from build123d import *

# Parameters (mm, degrees)
F0_W     = 20
F0_H     = 80
F1_DEPTH = 5
F3_W     = 5
F3_H     = 5
F3_R     = 0.75
F4_DEPTH = 10
F2_W     = 4.293
F2_H     = 4.31325
F2_R     = 0.75
F5_DEPTH = 5
F6_W     = 10
F6_H     = 20
F7_DEPTH = 30


with BuildPart() as f1:
    # F0 (on Front) → F1 (new body)
    with BuildSketch(Plane.XZ):
        Rectangle(F0_W, F0_H)
    extrude(amount=F1_DEPTH)

    # F3 (on Front) → F4 (join)
    with BuildSketch(Plane.XZ):
        with Locations((-0.917875, 18.532625)):
            Rectangle(F3_W, F3_H)
        with Locations((-0.917875, 18.532625)):
            Circle(F3_R, mode=Mode.SUBTRACT)
    extrude(amount=F4_DEPTH)

    # F2 (on face) → F5 (join)
    with BuildSketch(Plane.XZ.offset(5)):
        with Locations((-7.8535, -37.843375)):
            Rectangle(F2_W, F2_H)
        with Locations((-7.8535, -37.843375)):
            Circle(F2_R, mode=Mode.SUBTRACT)
    extrude(amount=F5_DEPTH)

    # F6 (on Front) → F7 (join)
    with BuildSketch(Plane.XZ):
        with Locations((15, 0)):
            Rectangle(F6_W, F6_H)
        Polygon((20, -10), (10, -10), (20, -20), align=None)
        Polygon((20, 20), (10, 10), (20, 10), align=None)
    extrude(amount=F7_DEPTH)


solid = f1.part
Source: CAD feature listing. Evaluate the final solid. Frame: model axes, mm. A direction names the side the tool comes from. Round coordinates to 2 decimals unless told otherwise and drop trailing zeros. Loops run counter-clockwise (first coordinate to the right, second up) from the corner with the lowest first, then second, coordinate; pieces in that order, holes last.
Q1. First-contact query: P1, Ø1.5, axis at x = -1, y = -6.5, coming from the -Z side; P2, Ø2.5, axis at y = -7.5, z = 17.5, coming from the -X side; P3, Ø2, axis at y = -6.5, z = -37, coming from the +X side. Flat tips, straight axial feed; report the tip coordinate or a pass-through.
Q2. Section A-A, the plane z = 14. Return loops of the section in (x, y), plus the area to 3 significant figures.
Q3. Mould query, pull axis X, two halves, no side actions, for faces 1 (the face through (10, -2, -25)), 2 (the face through (-1, -7, 21.033)), 3 (the face through (20, -15, 0)), 4 (the face through (10, -17, 0)). Classes: pulls with the +X half, pulls with the -X half, needs draft (parallel to the pull), parting line crosses it, or undercut.
Q4. Ray query, line 1 (X direction, y = -21.75, z = -7.5); line 2 (X direction, y = -7, z = -36); line 3 (Y direction, x = 9, z = -10.5). Return the intervals inside material, ascending.
Q5. Access query for faces 5 (the face through (-8, -7, -35.687)), 6 (the face through (1.582, -7, 18)), 7 (the face through (-5.707, -7, -38)), 8 (the face through (-7.51, -7.46, -38.51)), 9 (the face through (15, -15, -15)). Directions: +Z, -Z, +X, -X, +Y, -Y. A direction counts if a zero-diameter tool reaches every point of the face in a straight line with its end or side. Return the directions, or none.
Q6. Section D-D, the plane x = 2.5. Return loops of the section in (y, z), plus the area to 3 significant figures.
Q7. Section B-B, the plane y = -3.25. Return loops of the section in (x, z), plus the area to 3 significant figures.
Q8. Section C-C, the plane z = -6. Return loops of the section in (x, y).
Solutions:
1. P1: stops at z = 16.03
1. P2: stops at x = -3.42
1. P3: stops at x = -5.71
2. outline: (-10, -5) - (10, -5) - (10, 0) - (-10, 0) - close; (14, -30) - (20, -30) - (20, 0) - (14, 0) - close
2. area: 280 mm2
3. face 1: undercut
3. face 2: needs draft
3. face 3: pulls with the +X half
3. face 4: pulls with the -X half
4. line 1: x = 10 to 20
4. line 2: x = -10 to -5.71
4. line 3: y = -5 to 0
5. face 5: +Z, +X, -X, -Y
5. face 6: +Z, -Z, -Y
5. face 7: +Z, -Z, +X, -Y
5. face 8: -Y
5. face 9: -Z, +Y, -Y
6. outline: (-5, -40) - (0, -40) - (0, 40) - (-5, 40) - close
6. area: 400 mm2
7. outline: (-10, -40) - (10, -40) - (10, -10) - (20, -20) - (20, 20) - (10, 10) - (10, 40) - (-10, 40) - close
7. area: 1,900 mm2
8. outline: (-10, -5) - (10, -5) - (10, -30) - (20, -30) - (20, 0) - (-10, 0) - close
